```python
from build123d import *

# Parameters (mm, degrees)
F0_W     = 457.2
F0_H     = 1054.1
F1_DEPTH = 25.4
F2_W     = 279.4
F2_H     = 584.2
F3_DEPTH = 25.4
F5_DEPTH = 25.4


with BuildPart() as f1:
    # F0 (on Top) → F1 (new body)
    with BuildSketch(Plane.XY):
        with Locations((-45.277641, 104.469)):
            Rectangle(F0_W, F0_H)
    extrude(amount=F1_DEPTH)

    # F2 (on face) → F3 (join)
    with BuildSketch(Plane.XY.offset(25.4)):
        with Locations((-45.87521, 224.568032)):
            Rectangle(F2_W, F2_H)
    extrude(amount=F3_DEPTH)

    # F4 (on face) → F5 (cut)
    with BuildSketch(Plane.XY.offset(50.8)):
        with BuildLine():
            Line((-86.836747, 55.727709), (-86.836747, 17.627709))
            ThreePointArc((-86.836747, 17.627709), (-45.484862, -48.067084), (-10.636747, 21.297123))
            Line((-10.636747, 21.297123), (-10.636747, 55.727709))
            Line((-10.636747, 55.727709), (-86.836747, 55.727709))
        make_face()
        with BuildLine():
            Line((-84.68732, 183.664479), (-84.68732, 145.564479))
            ThreePointArc((-84.68732, 145.564479), (-43.335435, 79.869686), (-8.48732, 149.233893))
            Line((-8.48732, 149.233893), (-8.48732, 183.664479))
            Line((-8.48732, 183.664479), (-84.68732, 183.664479))
        make_face()
        with BuildLine():
            Line((-85.555011, 298.756876), (-85.555011, 260.656876))
            ThreePointArc((-85.555011, 260.656876), (-44.203125, 194.962082), (-9.355011, 264.32629))
            Line((-9.355011, 264.32629), (-9.355011, 298.756876))
            Line((-9.355011, 298.756876), (-85.555011, 298.756876))
        make_face()
        with BuildLine():
            Line((-85.304319, 406.970002), (-85.304319, 368.870002))
            ThreePointArc((-85.304319, 368.870002), (-43.952433, 303.175209), (-9.104319, 372.539416))
            Line((-9.104319, 372.539416), (-9.104319, 406.970002))
            Line((-9.104319, 406.970002), (-85.304319, 406.970002))
        make_face()
        with BuildLine():
            Line((-88.826308, 512.056686), (-88.826308, 473.956686))
            ThreePointArc((-88.826308, 473.956686), (-47.474423, 408.261893), (-12.626308, 477.6261))
            Line((-12.626308, 477.6261), (-12.626308, 512.056686))
            Line((-12.626308, 512.056686), (-88.826308, 512.056686))
        make_face()
    extrude(amount=-F5_DEPTH, mode=Mode.SUBTRACT)


solid = f1.part
```
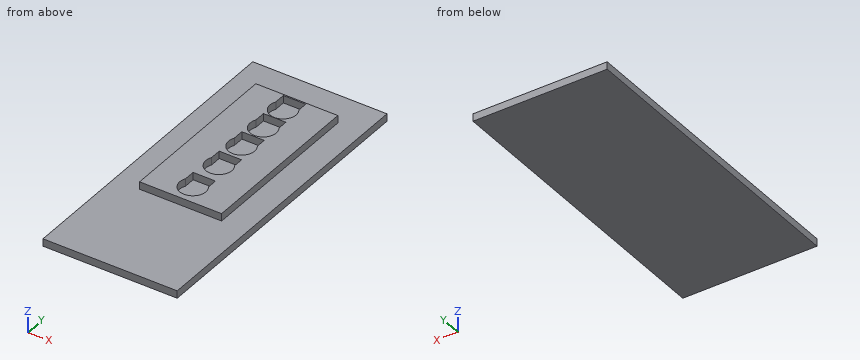
Geometry check sheet. Reference: the model listing, model coordinates, mm. Coordinates: 2 decimals unless noted, no trailing zeros. Write each loop counter-clockwise with the first axis right and the second up, starting at its lowest first coordinate (ties: lowest second). Pieces come first, ordered by that corner, then holes. Notation, with made-up numbers: M 0.5,14 L 16.5,14 A19 ccw 16.5,27 Z; hole C -4,88.25 d5. An arc over 180 degrees is marked long. One line per item, written item: value. Start each with the question number.
(1) Sectioned sample at B-B, the plane x = 44. Enter the section's corners in (y, z), and give its area (3 significant figures).
(2) Scan lines: line 1 along X through (y, z) = (395, 41); line 2 along Y through (x, z) = (-64, 40); line 3 along X through (y, z) = (294.5, 33.5). Record each from-to range of solid material in increasing order. Write a range as [from, to].
(3) Sectioned sample at A-A, the plane z = 40. Enter the section's corners in (x, y).
(4) Sectioned sample at D-D, the plane x = -26. Enter the section's corners in (y, z).
(5) Depth check by flat-ended pin: pin 1 (7.5 mm diameter, centred on y = 162, z = 43, fed in from -X); pin 2 (5 mm diameter, centred on x = 102.5, z = 27, fed in from +Y); pin 3 (7.5 mm diameter, centred on x = -44.5, z = 32.5, fed in from -Y); pin 4 (5 mm diameter, centred on x = -129.5, y = -306.5, fed in from +Z). Enter the tip coordinate at first touch or a pass-through.
(6) Sectioned sample at C-C, the plane y = -200. Enter the section's corners in (x, z), and give its area (3 significant figures).
Filled sheet:
1. outline: M -422.58,0 L 631.52,0 L 631.52,25.4 L 516.67,25.4 L 516.67,50.8 L -67.53,50.8 L -67.53,25.4 L -422.58,25.4 Z
1. area: 41,600 mm²
2. line 1: [-185.58, -85.3], [-9.1, 93.82]
2. line 2: [-67.53, -45], [55.73, 83.85], [183.66, 198.56], [298.76, 306.88], [406.97, 410.59], [512.06, 516.67]
2. line 3: [-185.58, -85.56], [-9.36, 93.82]
3. outline: M -185.58,-67.53 L 93.82,-67.53 L 93.82,516.67 L -185.58,516.67 Z; hole M -88.83,473.96 A44.56 ccw long -12.63,477.63 L -12.63,512.06 L -88.83,512.06 Z; hole M -86.84,17.63 A44.56 ccw long -10.64,21.3 L -10.64,55.73 L -86.84,55.73 Z; hole M -85.56,260.66 A44.56 ccw long -9.36,264.33 L -9.36,298.76 L -85.56,298.76 Z; hole M -85.3,368.87 A44.56 ccw long -9.1,372.54 L -9.1,406.97 L -85.3,406.97 Z; hole M -84.69,145.56 A44.56 ccw long -8.49,149.23 L -8.49,183.66 L -84.69,183.66 Z
4. outline: M -422.58,0 L 631.52,0 L 631.52,25.4 L 516.67,25.4 L 516.67,50.8 L 512.06,50.8 L 512.06,25.4 L 414.98,25.4 L 414.98,50.8 L 406.97,50.8 L 406.97,25.4 L 307.91,25.4 L 307.91,50.8 L 298.76,50.8 L 298.76,25.4 L 199.83,25.4 L 199.83,50.8 L 183.66,50.8 L 183.66,25.4 L 84.3,25.4 L 84.3,50.8 L 55.73,50.8 L 55.73,25.4 L -42.52,25.4 L -42.52,50.8 L -67.53,50.8 L -67.53,25.4 L -422.58,25.4 Z
5. pin 1: x = -185.58
5. pin 2: y = 631.52
5. pin 3: y = -67.53
5. pin 4: z = 25.4
6. outline: M -273.88,0 L 183.32,0 L 183.32,25.4 L -273.88,25.4 Z
6. area: 11,600 mm²
